```python
from build123d import *

# Parameters (mm, degrees)
F0_W      = 54
F0_H      = 29
F2_DEPTH  = 6
F1_W      = 42
F1_H      = 18
F3_DEPTH  = 25.4
F4_W      = 50
F4_H      = 25
F5_DEPTH  = 4
F6_W      = 10
F6_H      = 6
F7_DEPTH  = 5
F8_W      = 14
F8_H      = 10
F9_DEPTH  = 15
F10_W     = 12
F10_H     = 18.710866
F11_DEPTH = 8


with BuildPart() as f2:
    # F0 (on Top) → F2 (new body)
    with BuildSketch(Plane.XY):
        Rectangle(F0_W, F0_H)
    extrude(amount=F2_DEPTH)

    # F1 (on face) → F3 (cut)
    with BuildSketch(Plane.XY):
        with Locations((0, 1.5)):
            Rectangle(F1_W, F1_H)
    extrude(amount=F3_DEPTH, mode=Mode.SUBTRACT)

    # F4 (on face) → F5 (cut)
    with BuildSketch(Plane(origin=(0, 0, 0), x_dir=(1, 0, 0), z_dir=(0, 0, -1))):
        Rectangle(F4_W, F4_H)
    extrude(amount=-F5_DEPTH, mode=Mode.SUBTRACT)

    # F6 (on face) → F7 (cut)
    with BuildSketch(Plane.XZ.offset(14.5)):
        with Locations((1, 3)):
            Rectangle(F6_W, F6_H)
    extrude(amount=-F7_DEPTH, mode=Mode.SUBTRACT)

    # F8 (on face) → F9 (join)
    with BuildSketch(Plane.XZ.offset(14.5)):
        with Locations((1, 5)):
            Rectangle(F8_W, F8_H)
    extrude(amount=F9_DEPTH)

    # F10 (on face) → F11 (cut)
    with BuildSketch(Plane(origin=(0, 0, 0), x_dir=(1, 0, 0), z_dir=(0, 0, -1))):
        with Locations((1, 21.539463)):
            Rectangle(F10_W, F10_H)
    extrude(amount=-F11_DEPTH, mode=Mode.SUBTRACT)


solid = f2.part
```
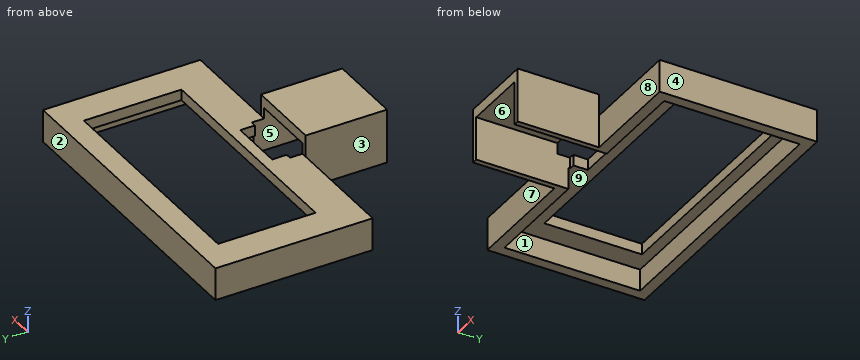
Here's how the part is built. I have some questions about the finished solid (model axes, mm). Face numbers are marked on the shaded views. A direction names the side the tool comes from. Give positions to 0.01 mm unless a question says otherwise; leave off trailing zeros. Write each loop counter-clockwise with the first axis right and the second up, starting at its lowest first coordinate (ties: lowest second). Pieces come first, ordered by that corner, then holes.
(1) Imagine slicing it at D-D, the plane x = -1. Write out the boundary of the cut face in (y, z), and give its area (3 significant figures).
Output values:
outline: (-29.5, 8) - (-14.5, 8) - (-14.5, 10) - (-29.5, 10) - close; (-9.5, 4) - (-7.5, 4) - (-7.5, 6) - (-9.5, 6) - close; (10.5, 4) - (12.5, 4) - (12.5, 0) - (14.5, 0) - (14.5, 6) - (10.5, 6) - close
area: 50.0 mm2
(2) Imagine slicing it at B-B, the plane x = 9. Write out the boundary of the cut face in (y, z).
Output values:
outline: (-14.5, 0) - (-12.5, 0) - (-12.5, 4) - (-7.5, 4) - (-7.5, 6) - (-14.5, 6) - close; (10.5, 4) - (12.5, 4) - (12.5, 0) - (14.5, 0) - (14.5, 6) - (10.5, 6) - close
(3) Imagine slicing it at A-A, the plane y = -4. Write out the boundary of the cut face in (x, z), and give its area (3 significant figures).
Output values:
outline: (-27, 0) - (-25, 0) - (-25, 4) - (-21, 4) - (-21, 6) - (-27, 6) - close; (21, 4) - (25, 4) - (25, 0) - (27, 0) - (27, 6) - (21, 6) - close
area: 40.0 mm2
(4) Will these pins go through, and if not, where does the flat tip stop? pin 1 (4 mm diameter, centred on x = -0.5, y = -11, fed in from -Z); pin 2 (2 mm diameter, centred on x = 20.5, y = -0.5, fed in from +Z); pin 3 (5 mm diameter, centred on y = -19, z = 4.5, fed in from -X).
Output values:
pin 1: stops at z = 4
pin 2: stops at z = 6
pin 3: stops at x = -6
(5) On a 3-axis mill with a long thin cutter (end or side, diameter ignored), from which of +Z, -Z, +X, -X, +Y, -Y can I reach the whole of each face in a straight line? I mean the marked faces 5, 6, 7, 8 and 9. Say none if no direction works.
Output values:
face 5: -Z, -Y
face 6: -Z, +Y, -Y
face 7: +Z, -Z, -X, -Y
face 8: +Z, -Z, +X, -Y
face 9: -Z
(6) Thinking about a two-plate mould opening in X: for the marked faces 1, 2, 3 and 4, which applies, pulls with the +X half, pulls with the -X half, needs draft (parallel to the pull), parting line crosses it, or undercut?
Output values:
face 1: undercut
face 2: needs draft
face 3: pulls with the -X half
face 4: pulls with the +X half
(7) If I drill on L1, parallel to X at y = 10.5, z = 3.25; L2, parallel to X at y = -18, z = 3; L3, parallel to Y at x = -5.5, z = 3, over which ranges is the centre line in solid material (lowest first)?
Output values:
L1: x = -27 to -25, 25 to 27
L2: x = -6 to -5, 7 to 8
L3: y = -29.5 to -12.5, 12.5 to 14.5
(8) Imagine slicing it at C-C, the plane z = 7.25. Write out the boundary of the cut face in (x, y).
Output values:
outline: (-6, -29.5) - (-5, -29.5) - (-5, -14.5) - (-6, -14.5) - close; (7, -29.5) - (8, -29.5) - (8, -14.5) - (7, -14.5) - close
